For this review, use the dimensioned drawing (mm, ordinates from the lowest corner) and the shaded views. A direction names the side the tool comes from. Round coordinates to 2 decimals unless told otherwise and drop trailing zeros. Order: outer loops, then holes, each group sorted by start corner. A loop starts at its lowest first (then second) coordinate and runs counter-clockwise, first axis right, second up. Notation, with made-up numbers: (-8.5, 28) - (14.5, 28) arc R19 ccw to (14.5, 35) - close; hole circle Ø2 at (82, -13). An arc over 180 degrees is marked (long way). Use CSV: the item, a comma, the result in double quotes. Start each with the question number.
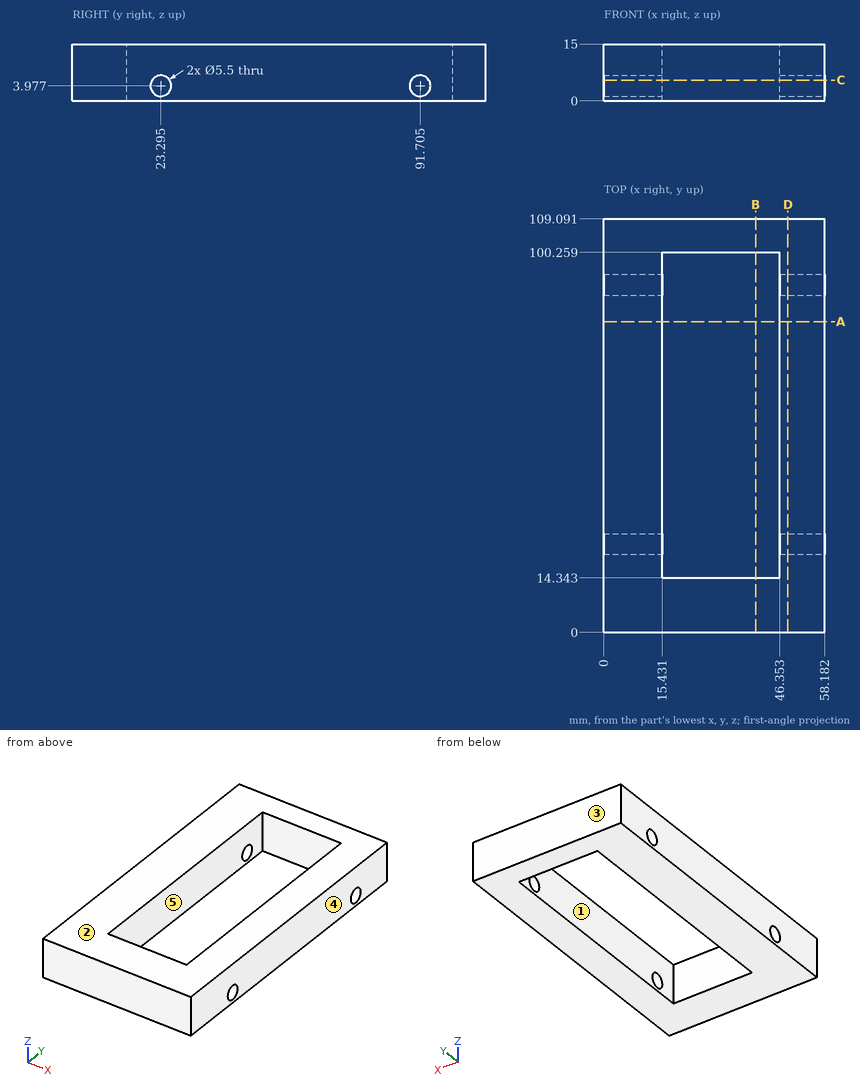
Q1. Clearance check with a flat-ended pin moving along its axis: pin 1 (3.5 mm diameter, centred on y = 91.7, z = 3.98, fed in from -X). State where the tip first meets the part, or that it passes through.
Q2. Tool access review of the marked faces 1 and 2: name each direction out of +Z, -Z, +X, -X, +Y, -Y from which nothing blocks a thin tool from reaching the whole face with its end or side.
Q3. Take a section at B-B (x = 40). State the section outline as (y, z) points.
Q4. The part is to be moulded in two halves that separate along X. For the marked faces 3, 4 and 5, say which applies: +X half, -X half, draft (parallel to the pull), parting line (faces both ways), or undercut.
Q5. Take a section at D-D (x = 48.5). Give the number of separate pieces and of enclosed holes in the cut face, plus the area to 3 significant figures.
Q6. For L1, parallel to X at y = 47, z = 11.25; L2, parallel to Y at x = 29.5, z = 3.5; L3, parallel to Y at x = 50.5, z = 3.5, list the stretches that pass through material, from the lowest coordinate up. Write a range as [from, to].
Q7. Take a section at C-C (z = 5.5). State the section outline as (x, y) points (1 decimal).
Q8. Take a section at A-A (y = 82). State the section outline as (x, z) points.
Findings below:
1,pin 1,"passes through"
2,face 1,"+Z, -Z"
2,face 2,"+Z, +X, -X, +Y, -Y"
3,outline,"(0, 0) - (14.34, 0) - (14.34, 15) - (0, 15) - close; (100.26, 0) - (109.09, 0) - (109.09, 15) - (100.26, 15) - close"
4,face 3,"draft"
4,face 4,"+X half"
4,face 5,"undercut"
5,separate pieces,"1"
5,enclosed holes,"2"
5,area,"1,590 mm^2"
6,L1,"x = [0, 15.43], [46.35, 58.18]"
6,L2,"y = [0, 14.34], [100.26, 109.09]"
6,L3,"y = [0, 20.59], [26, 89], [94.41, 109.09]"
7,outline,"(0, 0) - (58.2, 0) - (58.2, 21) - (46.4, 21) - (46.4, 14.3) - (15.4, 14.3) - (15.4, 21) - (0, 21) - close; (0, 25.6) - (15.4, 25.6) - (15.4, 89.4) - (0, 89.4) - close; (0, 94) - (15.4, 94) - (15.4, 100.3) - (46.4, 100.3) - (46.4, 94) - (58.2, 94) - (58.2, 109.1) - (0, 109.1) - close; (46.4, 25.6) - (58.2, 25.6) - (58.2, 89.4) - (46.4, 89.4) - close"
8,outline,"(0, 0) - (15.43, 0) - (15.43, 15) - (0, 15) - close; (46.35, 0) - (58.18, 0) - (58.18, 15) - (46.35, 15) - close"
